from build123d import *

# Parameters (mm, degrees)
SKETCH1_R           = 8.2
SKETCH1_R_2         = 6
SKETCH1_R_3         = 1.55
SKETCH1_W           = 3.1
SKETCH1_H           = 20
SKETCH1_W_2         = 5
SKETCH1_H_2         = 5
BOSS_EXTRUDE1_DEPTH = 5


with BuildPart() as part:
    # Sketch1 → Boss-Extrude1 (new body)
    with BuildSketch(Plane(origin=(0, 0, 0), x_dir=(1, 0, 0), z_dir=(0, 1, 0))):
        Polygon((-81.8, -30), (-66, -30), (-66, -35.1), (-51, -35.1), (-51, -30), (-30, -30), (-30, -35.1), (0, -35.1), (0, -30), (21, -30), (21, -35.1), (36, -35.1), (36, -30), (51.8, -30), (51.8, -18), (56.9, -18), (56.9, -6), (51.8, -6), (51.8, 6), (56.9, 6), (56.9, 18), (51.8, 18), (51.8, 30), (36, 30), (36, 35.1), (21, 35.1), (21, 30), (0, 30), (0, 35.1), (-30, 35.1), (-30, 30), (-51, 30), (-51, 35.1), (-66, 35.1), (-66, 30), (-81.8, 30), (-81.8, 18), (-86.9, 18), (-86.9, 6), (-81.8, 6), (-81.8, -6), (-86.9, -6), (-86.9, -18), (-81.8, -18), align=None)
        with Locations(Location((-4, -16, 0), (0, 0, 270))):
            Circle(SKETCH1_R, mode=Mode.SUBTRACT)
        with Locations(Location((-26, -16, 0), (0, 0, 270))):
            Circle(SKETCH1_R, mode=Mode.SUBTRACT)
        with Locations(Location((-15, 10, 0), (0, 0, 270))):
            Circle(SKETCH1_R_2, mode=Mode.SUBTRACT)
        with Locations(Location((5, -8.5, 0), (0, 0, 270))):
            Circle(SKETCH1_R_3, mode=Mode.SUBTRACT)
        with Locations(Location((5, -23.5, 0), (0, 0, 270))):
            Circle(SKETCH1_R_3, mode=Mode.SUBTRACT)
        with Locations(Location((-35, -8.5, 0), (0, 0, 270))):
            Circle(SKETCH1_R_3, mode=Mode.SUBTRACT)
        with Locations(Location((-35, -23.5, 0), (0, 0, 270))):
            Circle(SKETCH1_R_3, mode=Mode.SUBTRACT)
        with Locations(Location((-73.9, -13, 0), (0, 0, 270))):
            Circle(SKETCH1_R_3, mode=Mode.SUBTRACT)
        with Locations(Location((-60.9, -13, 0), (0, 0, 270))):
            Circle(SKETCH1_R_3, mode=Mode.SUBTRACT)
        with Locations(Location((30.9, -13, 0), (0, 0, 90))):
            Circle(SKETCH1_R_3, mode=Mode.SUBTRACT)
        with Locations(Location((43.9, -13, 0), (0, 0, 90))):
            Circle(SKETCH1_R_3, mode=Mode.SUBTRACT)
        with Locations((6.55, 10)):
            Rectangle(SKETCH1_W, SKETCH1_H, mode=Mode.SUBTRACT)
        with Locations((-36.55, 10)):
            Rectangle(SKETCH1_W, SKETCH1_H, mode=Mode.SUBTRACT)
        with Locations((-67.4, -7)):
            Rectangle(SKETCH1_W_2, SKETCH1_H_2, mode=Mode.SUBTRACT)
        with Locations((37.4, -7)):
            Rectangle(SKETCH1_W_2, SKETCH1_H_2, mode=Mode.SUBTRACT)
    extrude(amount=BOSS_EXTRUDE1_DEPTH)


solid = part.part
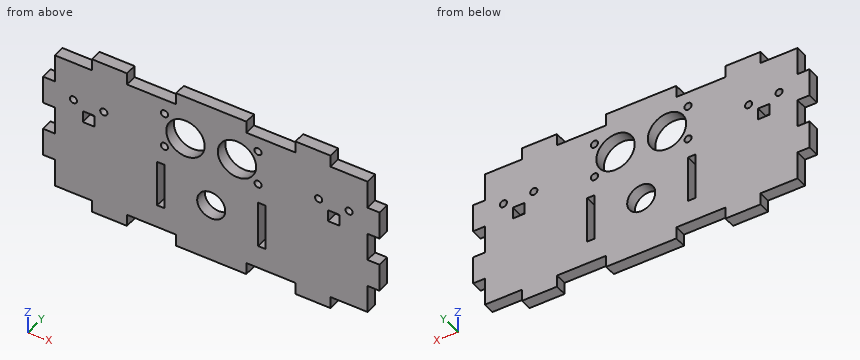
Here's how the part is built. I have some questions about the finished solid (model axes, mm). Coordinates: 2 decimals unless noted, no trailing zeros. Order: outer loops, then holes, each group sorted by start corner. A loop starts at its lowest first (then second) coordinate and runs counter-clockwise, first axis right, second up. Notation, with made-up numbers: (47.5, 43.25) - (76.5, 43.25) arc R14 ccw to (76.5, 62.25) - close; hole circle Ø9 at (-37, -24). An arc over 180 degrees is marked (long way). Use CSV: the item, a comma, the result in double quotes. Start each with the question number.
1. Suppose I cut it at A-A on x = -60.9. List the corners of the cut face in (y, z) for me, then the cut area to 4 significant figures.
2. Please list where these lines run through material, in increasing order: line 1 (X direction, y = 2.2, z = 16); line 2 (X direction, y = 2.45, z = -9.5); line 3 (Z direction, x = -69, y = 4.4). Write a range as from..to.
3. I'm going to push flat-ended pins straight in: pin 1 (1.5 mm diameter, centred on x = 53, y = 2.5, fed in from -Z); pin 2 (0.9 mm diameter, centred on x = -36, y = 3, fed in from +Z); pin 3 (1.5 mm diameter, centred on y = 2, z = 33, fed in from +X). Where does each tip first touch, or does it pass through?
4. Suppose I cut it at C-C on y = 3.05. Give the number of separate pieces and of enclosed holes in the cut face, then the cut area to 3 significant figures.
5. Suppose I cut it at B-B on z = -10. List the corners of the cut face in (x, y) for me, then the cut area to 3 significant figures.
Output:
1,outline,"(0, -35.1) - (5, -35.1) - (5, 11.45) - (0, 11.45) - close; (0, 14.55) - (5, 14.55) - (5, 35.1) - (0, 35.1) - close"
1,area,"335.5 mm2"
2,line 1,"x = -86.9..-34.2, -17.8..-12.2, 4.2..56.9"
2,line 2,"x = -86.9..-38.1, -35..-20.98, -9.02..5, 8.1..56.9"
2,line 3,"z = -30..4.5, 9.5..30"
3,pin 1,"stops at z = -18"
3,pin 2,"stops at z = 30"
3,pin 3,"stops at x = 36"
4,separate pieces,"1"
4,enclosed holes,"15"
4,area,"8,100 mm2"
5,outline,"(-86.9, 0) - (-38.1, 0) - (-38.1, 5) - (-86.9, 5) - close; (-35, 0) - (-21, 0) - (-21, 5) - (-35, 5) - close; (-9, 0) - (5, 0) - (5, 5) - (-9, 5) - close; (8.1, 0) - (56.9, 0) - (56.9, 5) - (8.1, 5) - close"
5,area,"628 mm2"
